Geometry: final body of the model. Coordinates: model frame, mm. A direction names the side the tool comes from. Round coordinates to 2 decimals unless told otherwise and drop trailing zeros. Loops run counter-clockwise (first coordinate to the right, second up) from the corner with the lowest first, then second, coordinate; pieces in that order, holes last. Notation, with made-up numbers: M 85.25,74.5 L 122.25,74.5 A16 cw 122.25,81.5 Z; hole C -16.75,-34 d7. An arc over 180 degrees is marked long. Write each question's results on one line, items separated by ' | '.
```python
from build123d import *

# Parameters (mm, degrees)
SKETCH1_W               = 90
SKETCH1_H               = 30
BOSS_EXTRUDE1_DEPTH     = 30
SHELL1_T                = -5
CUT_EXTRUDE1_DEPTH      = 100.498743711
CUT_EXTRUDE1_DEPTH_BACK = 100.498743711
SKETCH2_R               = 3
RIB1_REACH              = 101.499
SKETCH4_WALL_W          = 228.240511764
SKETCH4_WALL_H          = 6
MIRROR2_COPY_1_REACH    = 101.499
MIRROR2_COPY_1_SKETCH_W = 228.240511764
MIRROR2_COPY_1_SKETCH_H = 6


with BuildPart() as part:
    # Sketch1 → Boss-Extrude1 (new body)
    with BuildSketch(Plane(origin=(0, 0, 0), x_dir=(1, 0, 0), z_dir=(0, 1, 0))):
        with Locations((45, 15)):
            Rectangle(SKETCH1_W, SKETCH1_H)
    extrude(amount=BOSS_EXTRUDE1_DEPTH)

    # Shell1
    shell1_openings = [part.faces().sort_by_distance(p)[0] for p in [
        (45, 30, -15),
        (45, 15, -30),
        (45, 15, 0),
    ]]
    offset(amount=SHELL1_T, openings=shell1_openings, kind=Kind.INTERSECTION)

    # Sketch2 → Cut-Extrude1 (cut, two sides: drawn at the far end of the back side and taken through both)
    with BuildSketch(Plane(origin=(90, 0, 0), x_dir=(0, 0, -1), z_dir=(1, 0, 0)).offset(-CUT_EXTRUDE1_DEPTH_BACK)):
        with Locations((15, 22)):
            Circle(SKETCH2_R)
    extrude(amount=CUT_EXTRUDE1_DEPTH + CUT_EXTRUDE1_DEPTH_BACK, mode=Mode.SUBTRACT)

    # Sketch4 wall → Rib1 (add, up to next)
    with BuildSketch(Plane(origin=(10.412540423, 17.5, 0), x_dir=(0.397352390435, -0.917666103665, 0), z_dir=(0.917666103665, 0.397352390435, 0)), mode=Mode.PRIVATE) as rib1_sk1:
        with Locations((0, 3)):
            Rectangle(SKETCH4_WALL_W, SKETCH4_WALL_H)
    rib1_tool1 = extrude(rib1_sk1.sketch, amount=-RIB1_REACH, mode=Mode.PRIVATE) - part.part
    rib1 = rib1_tool1.solids().sort_by_distance((10.412540423, 17.5, 0))[0]
    add(rib1)

    # Mirror1: Rib1 across plane
    add(rib1.mirror(Plane(origin=(45, 0, 0), x_dir=(0, 0, 1), z_dir=(1, 0, 0))))

    # Mirror2: Rib1 across plane
    add(rib1.mirror(Plane.XY.offset(-15)))

    # Mirror2 copy 1 sketch → Mirror2 copy 1 (add, up to next)
    with BuildSketch(Plane(origin=(79.587459577, 17.5, -30), x_dir=(-0.397352390435, -0.917666103665, 0), z_dir=(-0.917666103665, 0.397352390435, 0)), mode=Mode.PRIVATE) as mirror2_copy_1_sk1:
        with Locations((0, 3)):
            Rectangle(MIRROR2_COPY_1_SKETCH_W, MIRROR2_COPY_1_SKETCH_H)
    mirror2_copy_1_tool1 = extrude(mirror2_copy_1_sk1.sketch, amount=-MIRROR2_COPY_1_REACH, mode=Mode.PRIVATE) - part.part
    add(mirror2_copy_1_tool1.solids().sort_by_distance((79.587459577, 17.5, -30))[0])


solid = part.part
```
1. Access query for faces 1 (the face through (48, 4, -30)), 2 (the face through (82, 13, -24)), 3 (the face through (10.337, 17.675, -3.042)). Directions: +Z, -Z, +X, -X, +Y, -Y. A direction counts if a zero-diameter tool reaches every point of the face in a straight line with its end or side. Return the directions, or none.
Answer key:
face 1: -Z, +X, -X, +Y, -Y | face 2: +Y | face 3: +Z, -Z, +Y
2. Section B-B (y = 13.5). Output: boundary loops of the cut face in (x, z).
Answer key:
outline: M 0,-30 L 12.14,-30 L 12.14,-24 L 5,-24 L 5,-6 L 12.14,-6 L 12.14,0 L 0,0 Z; M 77.86,-30 L 90,-30 L 90,0 L 77.86,0 L 77.86,-6 L 85,-6 L 85,-24 L 77.86,-24 Z
3. Ray query, probe 1 along Z at (x, y) = (88.3, 22); probe 2 along X at (y, z) = (5.5, -19.5); probe 3 along Y at (x, z) = (1.35, -15). Return the intervals inside material, ascending.
Answer key:
probe 1: z = -30 to -18, -12 to 0 | probe 2: x = 0 to 5, 85 to 90 | probe 3: y = 0 to 19, 25 to 30
4. Draft query along Y for faces 4 (the face through (8, 13, -24)), 5 (the face through (44, 0, -15)), 6 (the face through (2.5, 20.2, -12.6)), 7 (the face through (44, 5, -15)). Return one class per face: pulls with the +Y half, pulls with the -Y half, needs draft (parallel to the pull), parting line crosses it, or undercut.
Answer key:
face 4: needs draft | face 5: pulls with the -Y half | face 6: undercut | face 7: pulls with the +Y half
5. Pin query (flat end, axial travel): P1, Ø1, axis at y = 3, z = -22.5, coming from the -X side; P2, Ø12, axis at x = 20.5, z = -6, coming from the +Y side; P3, Ø4, axis at x = 73, z = -19.5, coming from the +Y side. Return the tip coordinate at first contact, or that it passes through.
Answer key:
P1: stops at x = 0 | P2: stops at y = 8.06 | P3: stops at y = 5
6. Section A-A (z = -15). Output: boundary loops of the cut face in (x, y).
Answer key:
outline: M 0,0 L 90,0 L 90,19 L 85,19 L 85,5 L 5,5 L 5,19 L 0,19 Z; M 0,25 L 5,25 L 5,30 L 0,30 Z; M 85,25 L 90,25 L 90,30 L 85,30 Z
7. Section D-D (x = 77). Output: boundary loops of the cut face in (y, z), then the cut area to 3 significant figures.
Answer key:
outline: M 0,-30 L 11.52,-30 L 11.52,-24 L 5,-24 L 5,-6 L 11.52,-6 L 11.52,0 L 0,0 Z | area: 228 mm²
8. Section C-C (y = 22). Output: boundary loops of the cut face in (x, z).
Answer key:
outline: M 0,-30 L 8.46,-30 L 8.46,-24 L 5,-24 L 5,-18 L 0,-18 Z; M 0,-12 L 5,-12 L 5,-6 L 8.46,-6 L 8.46,0 L 0,0 Z; M 81.54,-30 L 90,-30 L 90,-18 L 85,-18 L 85,-24 L 81.54,-24 Z; M 81.54,-6 L 85,-6 L 85,-12 L 90,-12 L 90,0 L 81.54,0 Z
